from build123d import *

# Parameters (mm, degrees)
EXTRUDE1_DEPTH = 0.45
FILLET2_START  = -0.45
FILLET2_DEPTH  = 0.9
FILLET1_R      = 0.544
SCALE1_SCALE   = 0.8


with BuildPart() as part:
    # Sketch1 → Extrude1 (new, symmetric)
    with BuildSketch(Plane(origin=(0, 0, 0), x_dir=(0, 0, -1), z_dir=(1, 0, 0))):
        with BuildLine():
            Line((-5.472300811, -4.20284711), (-1.929663183, -2.92))
            ThreePointArc((-1.929663183, -2.92), (-1.007472084, -3.351865152), (0, -3.5))
            Line((0, -3.5), (0, -5.367741935))
            ThreePointArc((0, -5.367741935), (3.203041928, -4.30733977), (5.140556326, -1.545100044))
            Line((5.140556326, -1.545100044), (3.351865152, -1.007472084))
            ThreePointArc((3.351865152, -1.007472084), (3.5, 0), (3.351865152, 1.007472084))
            Line((3.351865152, 1.007472084), (5.140556326, 1.545100044))
            ThreePointArc((5.140556326, 1.545100044), (3.203041928, 4.30733977), (0, 5.367741935))
            Line((0, 5.367741935), (0, 3.5))
            ThreePointArc((0, 3.5), (-1.007472084, 3.351865152), (-1.929663183, 2.92))
            Line((-1.929663183, 2.92), (-5.472300811, 4.20284711))
            ThreePointArc((-5.472300811, 4.20284711), (6.9, 0), (-5.472300811, -4.20284711))
        make_face()
    extrude(amount=EXTRUDE1_DEPTH, both=True)

    # Fillet2: read off the stored shape, not the designer's step
    # Fillet2 outline → Fillet2 (cut)
    with BuildSketch(Plane.YZ.offset(FILLET2_START)):
        with BuildLine():
            Line((-1.007472084, -3.351865152), (-1.35481354, -4.507472084))
            add(Edge.make_bspline(
                [(-1.35481354, -4.507472084), (-1.184355647, -3.940357738), (-0.701331375, -3.5), (0, -3.5)],
                knots=[0, 0, 0, 0, 0.5, 0.5, 0.5, 0.5], degree=3, weights=[1, 0.762616389, 0.643924583, 0.643924583]))
            ThreePointArc((0, -3.5), (-0.509152219, -3.462768259), (-1.007472084, -3.351865152))
        make_face()
        with BuildLine():
            ThreePointArc((1.007472084, -3.351865152), (0.509152221, -3.462768259), (2e-09, -3.5))
            add(Edge.make_bspline(
                [(2e-09, -3.5), (0.701331375, -3.5), (1.184355647, -3.940357738), (1.35481354, -4.507472084)],
                knots=[0.5, 0.5, 0.5, 0.5, 1, 1, 1, 1], degree=3, weights=[0.643924583, 0.643924583, 0.762616389, 1]))
            Line((1.35481354, -4.507472084), (1.007472084, -3.351865152))
        make_face()
    extrude(amount=FILLET2_DEPTH, mode=Mode.SUBTRACT)

    # Fillet1
    fillet1_edges = [part.edges().sort_by_distance(p)[0] for p in [
        (0, -5.367741935, 0),
        (0, 5.367741935, 0),
        (0, -4.20284711, 5.472300811),
        (0, 4.20284711, 5.472300811),
        (0, -1.545100044, -5.140556326),
        (0, 1.545100044, -5.140556326),
    ]]
    fillet(fillet1_edges, radius=FILLET1_R)


with BuildPart() as part_1:
    # Scale1: scaled about (0, 0, -1.222397064)
    add(part.part.scale(SCALE1_SCALE).moved(Location((0, 0, -0.244479413))))


solid = part_1.part
Design review of the part built by this model. Coordinates are the model's own, in mm. A direction names the side the tool comes from. Coordinates: 2 decimals unless noted, no trailing zeros. Loops run counter-clockwise (first coordinate to the right, second up) from the corner with the lowest first, then second, coordinate; pieces in that order, holes last. Notation, with made-up numbers: (-36, 8) - (5, 8) arc R25 cw to (5, 34) - close; hole circle Ø6 at (22.5, -38). An arc over 180 degrees is marked (long way). Use CSV: the item, a comma, the result in double quotes. Start each with the question number.
1. Add section A-A on y = 4. Give the boundary of the cut face in (x, z), plus the area to 3 significant figures.
2. Add section B-B on z = 0. Give the boundary of the cut face in (x, y).
3. For faces 1 (the flat face through (0.36, 0.1, -3.2)), 2 (the cylindrical face through (0.01, 3.43, -2.83)), 3 (the flat face through (0.005, -2.747, 2.434)), list the 3-axis set-ups (+Z, -Z, +X, -X, +Y, -Y) from which the entire face can be reached by the end or side of a thin tool; tool diameter is ignored.
4. To check wall thickness, follow probe 1 along Y at (x, z) = (-0.2, -4); probe 2 along Y at (x, z) = (0.1, -1.5); probe 3 along Y at (x, z) = (0, 3.75). State the ranges of each line that lie inside material, in increasing order.
5. Add section C-C on z = -4.5. Give the boundary of the cut face in (x, y).
Resolved:
1,outline,"(-0.36, -4.05) - (0.36, -4.05) - (0.36, -1.81) - (-0.36, -1.81) - close; (-0.36, -0.28) - (0.36, -0.28) - (0.36, 3.56) - (-0.36, 3.56) - close"
1,area,"4.38 mm2"
2,outline,"(-0.36, -5.51) - (0.36, -5.51) - (0.36, -2.79) - (-0.36, -2.79) - close; (-0.36, 2.79) - (0.36, 2.79) - (0.36, 5.51) - (-0.36, 5.51) - close"
3,face 1,"+Z, -Z, +X, +Y, -Y"
3,face 2,"+X, -X"
3,face 3,"+Z, +X, -X"
4,probe 1,"-4.05 to -2.08, -1.14 to 1.14, 2.08 to 4.05"
4,probe 2,"-5.38 to -4.11, 4.11 to 5.38"
4,probe 3,"-3.8 to -3.31, 3.31 to 3.8"
5,outline,"(-0.36, -3.52) - (0.36, -3.52) - (0.36, 3.52) - (-0.36, 3.52) - close"
